from build123d import *

# Parameters (mm, degrees)
F0_W      = 50
F0_H      = 43
F0_R      = 1.5
F1_DEPTH  = 78
F3_T      = -2
F2_R      = 11
F4_DEPTH  = 3.1
F5_R      = 3
F6_R      = 1.5
F7_DEPTH  = 75
F8_DEPTH  = 40
F9_W      = 50
F9_H      = 23
F10_DEPTH = 30


# Not quite as in the source:
# - a feature names something its author has since deleted; it is built from what else it names


with BuildPart() as f1:
    # F0 (on Top) → F1 (new body)
    with BuildSketch(Plane.XY):
        with Locations((-9.0278687937, 4.7237686813)):
            Rectangle(F0_W, F0_H)
        with Locations((-31.0278687937, -13.7762313187)):
            Circle(F0_R, mode=Mode.SUBTRACT)
        with Locations((12.9721312063, -13.7762313187)):
            Circle(F0_R, mode=Mode.SUBTRACT)
        with Locations((-31.0278687937, 23.2237686813)):
            Circle(F0_R, mode=Mode.SUBTRACT)
        with Locations((12.9721312063, 23.2237686813)):
            Circle(F0_R, mode=Mode.SUBTRACT)
        with Locations((12.9721312063, 23.2237686813)):
            Circle(F0_R)
        with Locations((12.9721312063, -13.7762313187)):
            Circle(F0_R)
        with Locations((-31.0278687937, -13.7762313187)):
            Circle(F0_R)
        with Locations((-31.0278687937, 23.2237686813)):
            Circle(F0_R)
    extrude(amount=F1_DEPTH)

    # F3
    f3_openings = [f1.faces().sort_by_distance(p)[0] for p in [
        (-9.027869, 4.723769, 0),
    ]]
    offset(amount=F3_T, openings=f3_openings)

    # F2 (on face) → F4 (cut)
    with BuildSketch(Plane.XY.offset(78)):
        with Locations((-9.0278687937, 4.7237686813)):
            Circle(F2_R)
    extrude(amount=-F4_DEPTH, mode=Mode.SUBTRACT)

    # F5
    f5_edges = [f1.edges().sort_by_distance(p)[0] for p in [
        (15.972131, 26.223769, 39),
        (-9.027869, 26.223769, 78),
        (-34.027869, 26.223769, 39),
        (15.972131, -16.776231, 39),
        (-9.027869, -16.776231, 78),
        (-34.027869, -16.776231, 39),
    ]]
    fillet(f5_edges, radius=F5_R)

    # F6 (on face) → F7 (join)
    with BuildSketch(Plane.XY):
        with BuildLine():
            ThreePointArc((12.9721312104, -16.7762313187), (15.0934515513, -15.8975516608), (15.9721312063, -13.7762313187))
            ThreePointArc((15.9721312063, -13.7762313187), (10.8508108613, -11.6549109766), (12.9721312104, -16.7762313187))
        make_face()
        with Locations((12.9721312063, -13.7762313187)):
            Circle(F6_R, mode=Mode.SUBTRACT)
        with BuildLine():
            ThreePointArc((12.9721312063, 26.2237686813), (10.8508108627, 21.1024483377), (15.9721312063, 23.2237686813))
            ThreePointArc((15.9721312063, 23.2237686813), (15.0934515498, 25.3450890248), (12.9721312063, 26.2237686813))
        make_face()
        with Locations((12.9721312063, 23.2237686813)):
            Circle(F6_R, mode=Mode.SUBTRACT)
        with BuildLine():
            ThreePointArc((-34.0278687937, -13.776231286), (-33.1491891488, -15.8975516507), (-31.0278687937, -16.7762313187))
            ThreePointArc((-31.0278687937, -16.7762313187), (-28.9065484502, -15.8975516623), (-28.0278687937, -13.7762313187))
            ThreePointArc((-28.0278687937, -13.7762313187), (-31.0278687774, -10.7762313187), (-34.0278687937, -13.776231286))
        make_face()
        with Locations((-31.0278687937, -13.7762313187)):
            Circle(F6_R, mode=Mode.SUBTRACT)
        with BuildLine():
            ThreePointArc((-28.0278687937, 23.2237686813), (-28.9065484366, 25.3450890113), (-31.0278687555, 26.2237686813))
            ThreePointArc((-31.0278687555, 26.2237686813), (-33.1491891237, 25.3450890384), (-34.0278687937, 23.2237686813))
            ThreePointArc((-34.0278687937, 23.2237686813), (-31.0278687937, 20.2237686813), (-28.0278687937, 23.2237686813))
        make_face()
        with Locations((-31.0278687937, 23.2237686813)):
            Circle(F6_R, mode=Mode.SUBTRACT)
    extrude(amount=F7_DEPTH)

    # F0 (on Top) → F8 (cut)
    with BuildSketch(Plane.XY):
        with Locations((-31.0278687937, 23.2237686813)):
            Circle(F0_R)
        with Locations((12.9721312063, 23.2237686813)):
            Circle(F0_R)
        with Locations((-31.0278687937, -13.7762313187)):
            Circle(F0_R)
        with Locations((12.9721312063, -13.7762313187)):
            Circle(F0_R)
    extrude(amount=F8_DEPTH, mode=Mode.SUBTRACT)

    # F9 (on Top) → F10 (cut)
    with BuildSketch(Plane.XY):
        with Locations((-9.0278687937, 14.7237686813)):
            Rectangle(F9_W, F9_H)
    extrude(amount=F10_DEPTH, mode=Mode.SUBTRACT)


solid = f1.part
Geometry check sheet. Reference: the model listing, model coordinates, mm. A direction names the side the tool comes from. Round coordinates to 2 decimals unless told otherwise and drop trailing zeros. Order: outer loops, then holes, each group sorted by start corner. A loop starts at its lowest first (then second) coordinate and runs counter-clockwise, first axis right, second up. Notation, with made-up numbers: M 89.25,81.5 L 106.25,81.5 A10 cw 106.25,87.5 Z; hole C 85.25,75.5 d4. An arc over 180 degrees is marked long. Answer in a Markdown table with one row per item. Add a question column.
Item 1: Sectioned sample at C-C, the plane z = 34.5. Enter the section's corners in (x, y).
Item 2: Set-up check for faces 5 (the face through (12, -12, 75)), 6 (the face through (-17.135, 12.158, 77.014)), 7 (the face through (11.782, 22.311, 47.185)): record each of +Z, -Z, +X, -X, +Y, -Y from which the full face is reachable in a straight line by a thin tool's end or side.
Item 3: Draft check along Y on faces 1 (the face through (-30, -12, 75)), 2 (the face through (11, 22, 75)), 3 (the face through (-9, -16.776, 37)), 4 (the face through (15, 3.224, 15)). Enter one of: released by +Y, released by -Y, zero draft, split by the parting line, or undercut.
Item 4: Sectioned sample at A-A, the plane y = 10. Enter the section's corners in (x, z), plus the area to 3 significant figures.
Item 5: Depth check by flat-ended pin: pin 1 Ø2 at (x, z) = (-32.5, 12) entering from +Y; pin 2 Ø1.3 at (x, y) = (13.5, 24) entering from -Z; pin 3 Ø11.5 at (x, y) = (-12, 6) entering from -Z; pin 4 Ø2 at (x, y) = (-31, 23.5) entering from -Z. Enter the tip coordinate at first touch or a pass-through.
Item 6: Sectioned sample at B-B, the plane x = 4. Enter the section's corners in (y, z), plus the area to 3 significant figures.
Item 7: Material ranges on L1, parallel to Z at x = 12, y = -12; L2, parallel to Y at x = -18, z = 47; L3, parallel to X at y = 23, z = 60, recorded low to high. Write a range as [from, to].
Item 8: Sectioned sample at D-D, the plane y = -8.5. Enter the section's corners in (x, z).
Filled in:
| question | item | result |
|---|---|---|
| 1 | outline | M -34.03,-13.78 A3 ccw -31.03,-16.78 L 12.97,-16.78 A3 ccw 15.97,-13.78 L 15.97,23.22 A3 ccw 12.97,26.22 L -31.03,26.22 A3 ccw -34.03,23.22 Z; hole C -31.03,-13.78 d3; hole C -31.03,23.22 d3; hole M -32.03,-10.95 A3 cw -28.2,-14.78 L 10.14,-14.78 A3 cw 13.97,-10.95 L 13.97,20.4 A3 cw 10.14,24.22 L -28.2,24.22 A3 cw -32.03,20.4 Z; hole C 12.97,-13.78 d3; hole C 12.97,23.22 d3 |
| 2 | face 5 | none |
| 2 | face 6 | +Z, -Z |
| 2 | face 7 | -Z |
| 3 | face 1 | undercut |
| 3 | face 2 | undercut |
| 3 | face 3 | released by -Y |
| 3 | face 4 | released by +Y |
| 4 | outline | M -34.03,30 L -32.03,30 L -32.03,76 L -18.68,76 L -18.68,78 L -34.03,78 Z; M 0.62,76 L 13.97,76 L 13.97,30 L 15.97,30 L 15.97,78 L 0.62,78 Z |
| 4 | area | 245 mm² |
| 5 | pin 1 | stops at y = 3.22 |
| 5 | pin 2 | stops at z = 30 |
| 5 | pin 3 | passes through |
| 5 | pin 4 | stops at z = 40 |
| 6 | outline | M -16.78,0 L -14.78,0 L -14.78,76 L 24.22,76 L 24.22,30 L 26.22,30 L 26.22,75 A3 ccw 23.22,78 L -13.78,78 A3 ccw -16.78,75 Z |
| 6 | area | 326 mm² |
| 7 | L1 | z = [0, 75], [76, 78] |
| 7 | L2 | y = [-16.78, -14.78], [24.22, 26.22] |
| 7 | L3 | x = [-34.03, -32.03], [-29.54, -28.04], [9.98, 11.49], [13.97, 15.97] |
| 8 | outline | M -34.03,0 L -32.03,0 L -32.03,76 L 13.97,76 L 13.97,0 L 15.97,0 L 15.97,78 L -34.03,78 Z |
